```python
from build123d import *

# Parameters (mm, degrees)
SKETCH_1_W          = 10
SKETCH_1_H          = 3
EXTRUDE_1_DEPTH     = 10
SKETCH_2_R          = 2.2
CUT_EXTRUDE_1_DEPTH = 11
SKETCH_3_R          = 1.75
CUT_EXTRUDE_2_DEPTH = 4
FILLET_1_R          = 3
FILLET_2_R          = 1


with BuildPart() as part:
    # ｽｹｯﾁ1 → ﾎﾞｽ - 押し出し1 (new body)
    with BuildSketch(Plane.XY):
        Polygon((5, 10), (0, 10), (0, -5), (5, -5), (5, 7), align=None)
        with Locations((10, 8.5)):
            Rectangle(SKETCH_1_W, SKETCH_1_H)
        Polygon((0, -5), (0, 10), (-5, 10), (-5, 7), (-5, -5), align=None)
        with Locations((-10, 8.5)):
            Rectangle(SKETCH_1_W, SKETCH_1_H)
    extrude(amount=EXTRUDE_1_DEPTH)

    # ｽｹｯﾁ2 → ｶｯﾄ - 押し出し1 (cut, through all)
    with BuildSketch(Plane(origin=(0, 0, 0), x_dir=(-1, 0, 0), z_dir=(0, 0, -1))):
        Circle(SKETCH_2_R)
    extrude(amount=-CUT_EXTRUDE_1_DEPTH, mode=Mode.SUBTRACT)

    # ｽｹｯﾁ3 → ｶｯﾄ - 押し出し2 (cut, through all)
    with BuildSketch(Plane.XZ.offset(-7)):
        with Locations((-11.5, 5)):
            Circle(SKETCH_3_R)
        with Locations((11.5, 5)):
            Circle(SKETCH_3_R)
    extrude(amount=-CUT_EXTRUDE_2_DEPTH, mode=Mode.SUBTRACT)

    # ﾌｨﾚｯﾄ1
    fillet_1_edges = [part.edges().sort_by_distance(p)[0] for p in [
        (5, -5, 5),
        (-5, -5, 5),
        (-5, 7, 5),
        (5, 7, 5),
    ]]
    fillet(fillet_1_edges, radius=FILLET_1_R)

    # ﾌｨﾚｯﾄ2
    fillet_2_edges = [part.edges().sort_by_distance(p)[0] for p in [
        (-15, 8.5, 0),
        (15, 8.5, 0),
        (15, 8.5, 10),
        (-15, 7, 5),
        (15, 7, 5),
        (-15, 8.5, 10),
        (-5, 1, 0),
        (-5, 1, 10),
        (-11.5, 7, 0),
        (-11.5, 7, 10),
        (11.5, 7, 0),
        (11.5, 7, 10),
        (5, 1, 0),
        (5, 1, 10),
        (0, -5, 0),
        (0, -5, 10),
        (4.121320344, -4.121320344, 0),
        (-4.121320344, -4.121320344, 0),
        (4.121320344, -4.121320344, 10),
        (-4.121320344, -4.121320344, 10),
        (-5.878679656, 6.121320344, 0),
        (-5.878679656, 6.121320344, 10),
        (5.878679656, 6.121320344, 0),
        (5.878679656, 6.121320344, 10),
    ]]
    fillet(fillet_2_edges, radius=FILLET_2_R)


solid = part.part
```
Source: CAD feature listing. Evaluate the final solid. Frame: model axes, mm. A direction names the side the tool comes from. Round coordinates to 2 decimals unless told otherwise and drop trailing zeros. Loops run counter-clockwise (first coordinate to the right, second up) from the corner with the lowest first, then second, coordinate; pieces in that order, holes last. Notation, with made-up numbers: M 41.25,45.5 L 92.25,45.5 A24 ccw 92.25,67.5 Z; hole C 9.5,16 d10. An arc over 180 degrees is marked long. Put each result on its own line as item: value.
(1) Section A-A, the plane z = 5. Return loops of the section in (x, y), and give its area (3 significant figures).
Solutions:
outline: M -15,8 A1 ccw -14,7 L -13.25,7 L -13.25,10 L -15,10 Z; M -9.75,7 L -8,7 A3 cw -5,4 L -5,-2 A3 ccw -2,-5 L 2,-5 A3 ccw 5,-2 L 5,4 A3 cw 8,7 L 9.75,7 L 9.75,10 L -9.75,10 Z; M 13.25,7 L 14,7 A1 ccw 15,8 L 15,10 L 13.25,10 Z; hole C 0,0 d4.4
area: 173 mm²
(2) Section D-D, the plane y = 0. Return loops of the section in (x, z).
Solutions:
outline: M -5,1 A1 ccw -4,0 L -2.2,0 L -2.2,10 L -4,10 A1 ccw -5,9 Z; M 2.2,0 L 4,0 A1 ccw 5,1 L 5,9 A1 ccw 4,10 L 2.2,10 Z
(3) First-contact query: pin 1 (1 mm diameter, centred on x = -9.5, z = 6, fed in from -Y); pin 2 (5 mm diameter, centred on y = -0.5, z = 6.5, fed in from +X); pin 3 (5 mm diameter, centred on y = 1, z = 5, fed in from -X). Flat tips, straight axial feed; report the tip coordinate or a pass-through.
Solutions:
pin 1: y = 7
pin 2: x = 5
pin 3: x = -5
(4) Section C-C, the plane y = 8.5. Return loops of the section in (x, z).
Solutions:
outline: M -15,1 A1 ccw -14,0 L 14,0 A1 ccw 15,1 L 15,9 A1 ccw 14,10 L -14,10 A1 ccw -15,9 Z; hole C -11.5,5 d3.5; hole C 11.5,5 d3.5
(5) Pull-direction query (Z, two-part tool) for faces 1 (the face through (-10.958, 7.301, 0.285)), 2 (the face through (5, 1, 5)), 3 (the face through (14.699, 9.014, 9.715)), 4 (the face through (-10.69, 8.48, 3.45)); classes: released by +Z, released by -Z, zero draft, split by the parting line, or undercut.
Solutions:
face 1: released by -Z
face 2: zero draft
face 3: released by +Z
face 4: undercut
(6) Access query for faces 5 (the face through (9.6, 7, 4.9)), 6 (the face through (-4.699, 0.958, 0.285)), 7 (the face through (11.042, 7.301, 0.285)), 8 (the face through (-4.699, 0.958, 9.715)), 9 (the face through (-14.715, 7.301, 5.056)). Directions: +Z, -Z, +X, -X, +Y, -Y. A direction counts if a zero-diameter tool reaches every point of the face in a straight line with its end or side. Return the directions, or none.
Solutions:
face 5: +Z, -Z, +X, -Y
face 6: -Z, -X, -Y
face 7: -Z, +X, -Y
face 8: +Z, -X, -Y
face 9: +Z, -Z, -X, -Y
(7) Section B-B, the plane x = 0. Return loops of the section in (y, z).
Solutions:
outline: M -5,1 A1 ccw -4,0 L -2.2,0 L -2.2,10 L -4,10 A1 ccw -5,9 Z; M 2.2,0 L 10,0 L 10,10 L 2.2,10 Z
(8) Ray query, line 1 (Z direction, x = -11.5, y = 8.25); line 2 (Y direction, x = 0, z = 3.5); line 3 (X direction, y = 8, z = 5.5). Return the intervals inside material, ascending. Write a range as [from, to].
Solutions:
line 1: [0, 3.25], [6.75, 10]
line 2: [-5, -2.2], [2.2, 10]
line 3: [-15, -13.18], [-9.82, 9.82], [13.18, 15]
